Read the model definition and answer for the solid it produces. Units are mm, in the model's axes. Coordinates: 2 decimals unless noted, no trailing zeros. Loops run counter-clockwise (first coordinate to the right, second up) from the corner with the lowest first, then second, coordinate; pieces in that order, holes last. Notation, with made-up numbers: (32.25, -9) - (79.25, -9) arc R15 cw to (79.25, 6) - close; hole circle Ø4 at (8, 88). An arc over 180 degrees is marked (long way). One line per question, with ' | ' between items. Start each with the question number.
```python
from build123d import *

# Parameters (mm, degrees)
F0_W     = 150
F0_H     = 6
F1_DEPTH = 6
F2_W     = 6
F2_H     = 25
F3_DEPTH = 6


with BuildPart() as f1:
    # F0 (on Right) → F1 (new body)
    with BuildSketch(Plane.YZ):
        Polygon((-75, 25), (-150, 25), (-150, 12.5), (-144, 12.5), (-144, -12.5), (-150, -12.5), (-150, -25), (-75, -25), (-75, -19), (75, -19), (75, -25), (150, -25), (150, -12.5), (144, -12.5), (144, 12.5), (150, 12.5), (150, 25), (75, 25), (75, 19), (-75, 19), align=None)
        with Locations((0, 28)):
            Rectangle(F0_W, F0_H)
        with Locations((0, 22)):
            Rectangle(F0_W, F0_H)
        with Locations((0, -28)):
            Rectangle(F0_W, F0_H)
        with Locations((0, -22)):
            Rectangle(F0_W, F0_H)
    extrude(amount=F1_DEPTH)

    # F2 (on face) → F3 (cut, through all)
    with BuildSketch(Plane.YZ.offset(6)):
        with Locations((-50, 0)):
            Rectangle(F2_W, F2_H)
        with Locations((50, 0)):
            Rectangle(F2_W, F2_H)
    extrude(amount=-F3_DEPTH, mode=Mode.SUBTRACT)


solid = f1.part
```
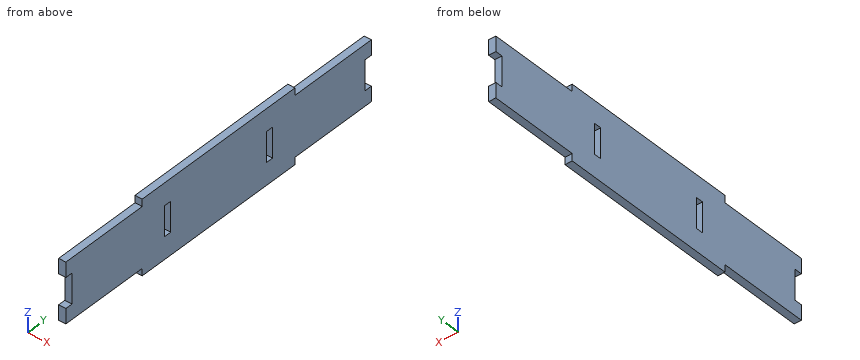
1) The part is cut by section A-A on x = 2.15. Write down the section's boundary in (y, z).
2) The part is cut by section C-C on y = -91.5. Write down the section's boundary in (x, z).
3) The part is cut by section B-B on z = -9. Write down the section's boundary in (x, y).
4) Given pin 1 Ø1.8 at (x, y) = (3, -119.5) entering from -Z; pin 2 Ø3 at (x, z) = (3.5, -3.5) entering from -Y; pin 3 Ø1.8 at (x, y) = (3, 146.5) entering from +Z, each flat-ended and moving along its own axis, determine where each tip first touches the part or whether it passes through.
5) Find the intervals of material crossed by line 1 along Y through (x, z) = (4.4, 5); line 2 along Z through (x, y) = (2.55, 52.5); line 3 along Z through (x, y) = (4.55, 100.5), in increasing order. Write a range as from..to.
Answer below:
1) outline: (-150, -25) - (-75, -25) - (-75, -31) - (75, -31) - (75, -25) - (150, -25) - (150, -12.5) - (144, -12.5) - (144, 12.5) - (150, 12.5) - (150, 25) - (75, 25) - (75, 31) - (-75, 31) - (-75, 25) - (-150, 25) - (-150, 12.5) - (-144, 12.5) - (-144, -12.5) - (-150, -12.5) - close; hole (-53, -12.5) - (-47, -12.5) - (-47, 12.5) - (-53, 12.5) - close; hole (47, -12.5) - (53, -12.5) - (53, 12.5) - (47, 12.5) - close
2) outline: (0, -25) - (6, -25) - (6, 25) - (0, 25) - close
3) outline: (0, -144) - (6, -144) - (6, -53) - (0, -53) - close; (0, -47) - (6, -47) - (6, 47) - (0, 47) - close; (0, 53) - (6, 53) - (6, 144) - (0, 144) - close
4) pin 1: z = -25 | pin 2: y = -144 | pin 3: z = 25
5) line 1: -144..-53, -47..47, 53..144 | line 2: -31..-12.5, 12.5..31 | line 3: -25..25
